from build123d import *

# Parameters (mm, degrees)
PAD017_DEPTH       = 15
SKETCH040_R        = 2
POCKET019_DEPTH    = 9.001
SKETCH_W           = 19.6
SKETCH_H           = 18.5
SKETCH_R           = 7.6
PAD_DEPTH          = 22
SKETCH002_W        = 17.1
SKETCH002_H        = 8.4
PAD001_DEPTH       = 8.5
POCKET_DEPTH       = 8
PAD002_DEPTH       = 13.6
SKETCH005_R        = 2
POCKET001_DEPTH    = 22.001
POCKET002_DEPTH    = 101.929968
POLARPATTERN_COUNT = 8
PAD004_DEPTH       = 1.5
SKETCH041_R        = 1.3
POCKET020_DEPTH    = 5


with BuildPart() as body023:
    # Sketch039 (on DatumPlane) → Pad017 (new body)
    with BuildSketch(Plane(origin=(0, -9.8, 0), x_dir=(0, 0, -1), z_dir=(0, -1, 0))):
        with BuildLine():
            Line((-9, 0), (-0.25, 0))
            Line((-0.25, 0), (-0.25, -6.907629))
            ThreePointArc((-0.25, -6.907629), (-4.1, -11), (-0.25, -15.092371))
            Line((-0.25, -15.092371), (-0.25, -22))
            Line((-0.25, -22), (-9, -22))
            Line((-9, -22), (-9, 0))
        make_face()
    extrude(amount=PAD017_DEPTH)

    # Sketch040 → Pocket019 (cut, through all)
    with BuildSketch(Plane.XY):
        with Locations((-18.546185, -20.8)):
            Circle(SKETCH040_R)
        with Locations((-18.546185, -13.8)):
            Circle(SKETCH040_R)
        with Locations((-3.453815, -13.8)):
            Circle(SKETCH040_R)
        with Locations((-3.453815, -20.8)):
            Circle(SKETCH040_R)
    extrude(amount=POCKET019_DEPTH, mode=Mode.SUBTRACT)


with BuildPart() as printable_axisholder_x_fusion:
    # Sketch → Pad (new body)
    with BuildSketch(Plane.YZ):
        with Locations((0, -0.25)):
            Rectangle(SKETCH_W, SKETCH_H)
        Circle(SKETCH_R, mode=Mode.SUBTRACT)
    extrude(amount=-PAD_DEPTH)

    # Sketch002 → Pad001 (join)
    with BuildSketch(Plane(origin=(0, 0, 9), x_dir=(0, -1, 0), z_dir=(0, 0, 1))):
        with Locations((-1.25, -17.8)):
            Rectangle(SKETCH002_W, SKETCH002_H)
    extrude(amount=PAD001_DEPTH)

    # Sketch003 → Pocket (cut)
    with BuildSketch(Plane(origin=(0, -7.3, 0), x_dir=(0, 0, -1), z_dir=(0, -1, 0))):
        with BuildLine():
            Line((-10.5, -22), (-10.5, -13.6))
            Line((-10.5, -13.6), (-11.6, -13.6))
            ThreePointArc((-12.1, -14.1), (-11.746447, -13.953553), (-11.6, -13.6))
            ThreePointArc((-12.1, -14.1), (-12.6, -14.6), (-12.1, -15.1))
            ThreePointArc((-12.1, -16.1), (-11.6, -15.6), (-12.1, -15.1))
            ThreePointArc((-12.1, -16.1), (-12.6, -16.6), (-12.1, -17.1))
            ThreePointArc((-12.1, -18.1), (-11.6, -17.6), (-12.1, -17.1))
            ThreePointArc((-12.1, -18.1), (-12.6, -18.6), (-12.1, -19.1))
            ThreePointArc((-12.1, -20.1), (-11.6, -19.6), (-12.1, -19.1))
            ThreePointArc((-12.1, -20.1), (-12.6, -20.6), (-12.1, -21.1))
            ThreePointArc((-11.8, -22), (-11.625658, -21.441886), (-12.1, -21.1))
            Line((-11.8, -22), (-10.5, -22))
        make_face()
    extrude(amount=-POCKET_DEPTH, mode=Mode.SUBTRACT)

    # Sketch004 (on DatumPlane) → Pad002 (join)
    with BuildSketch(Plane.YZ):
        Polygon((9.8, 17.5), (1.3, 17.5), (1.3, 16.25), (8.55, 16.25), (8.55, 9), (9.8, 9), align=None)
    extrude(amount=-PAD002_DEPTH)

    # Sketch005 (on DatumPlane) → Pocket001 (cut, through all)
    with BuildSketch(Plane.YZ):
        with Locations((4, 12.625)):
            Circle(SKETCH005_R)
    extrude(amount=-POCKET001_DEPTH, mode=Mode.SUBTRACT)

    # Sketch006 (on DatumPlane) → Pocket002 (cut, through all)
    with BuildSketch(Plane.YZ):
        with BuildLine():
            ThreePointArc((-7.846282, 1.560723), (-8, 0), (-7.846282, -1.560723))
            Line((-6.708571, -1.334418), (-7.846282, -1.560723))
            ThreePointArc((-6.708571, 1.334418), (-6.84, 0), (-6.708571, -1.334418))
            Line((-6.708571, 1.334418), (-7.846282, 1.560723))
        make_face()
    pocket002 = extrude(amount=-POCKET002_DEPTH, mode=Mode.SUBTRACT)

    # PolarPattern: Pocket002 ×8 about axis
    polarpattern_axis = Axis((0, 0, 0), (1, 0, 0))
    for i in range(1, POLARPATTERN_COUNT):
        add(pocket002.rotate(polarpattern_axis, i * 360 / POLARPATTERN_COUNT), mode=Mode.SUBTRACT)

    # Sketch010 (on DatumPlane) → Pad004 (join)
    with BuildSketch(Plane.XY.offset(9)):
        Polygon((0, -7.8), (-13.6, -7.8), (-13.6, -7.3), (-22, -7.3), (-22, -9.8), (0, -9.8), align=None)
    extrude(amount=PAD004_DEPTH)

    # Sketch041 → Pocket020 (cut)
    with BuildSketch(Plane.XY.offset(-9.5)):
        with Locations((-11, 0)):
            Circle(SKETCH041_R)
    extrude(amount=POCKET020_DEPTH, mode=Mode.SUBTRACT)

    # Fusion: union Body023
    add(body023.part)


solid = printable_axisholder_x_fusion.part
Work out the finished part from the listing and answer in its coordinate system (mm). A direction names the side the tool comes from. Coordinates: 2 decimals unless noted, no trailing zeros. Order: outer loops, then holes, each group sorted by start corner. A loop starts at its lowest first (then second) coordinate and runs counter-clockwise, first axis right, second up. Notation, with made-up numbers: (28.25, 23) - (41.25, 23) arc R33 cw to (41.25, 53) - close; hole circle Ø1 at (-11, 7.25). An arc over 180 degrees is marked (long way). Put each result on its own line as item: value. Start each with the question number.
1) Find the intervals of material crossed by line 1 (X direction, y = -20.8, z = 7); line 2 (Y direction, x = -11, z = -8.45); line 3 (Z direction, x = -16.75, y = 4) (3 decimals), in increasing order. Write a range as from..to.
2) Find section B-B (z = -3.75). Give the vertices of the cut face in (x, y).
3) Find section D-D (y = -17). Give the vertices of the cut face in (x, z).
4) For a pull along X with two mould halves and no side action, classify faces 4 (the cylindrical face through (-10.846, 7.013, -2.928)), 5 (the cylindrical face through (-10.9, -17.2, 4.1)) as released by +X, released by -X, zero draft, split by the parting line, or undercut.
5) For faces 1 (the flat face through (-7, 0, 9)), 2 (the cylindrical face through (-10.846, -7.013, 2.928)), 3 (the flat face through (-11, -24.8, 5)), determine the directions among +Z, -Z, +X, -X, +Y, -Y from which every point of the face is accessible in a straight line to the end or side of a thin tool.
6) Find section C-C (y = -5). Give the vertices of the cut face in (x, z) (3 decimals), plus the area to 3 significant figures.
7) Find section A-A (z = 3.5). Give the vertices of the cut face in (x, y).
8) Flat-ended cylindrical pins translate along their axes: pin 1 (3.5 mm diameter, centred on x = -3.45, y = -20.8, fed in from +Z) (3 decimals); pin 2 (5 mm diameter, centred on x = -9, y = -20.5, fed in from -Z); pin 3 (1.4 mm diameter, centred on x = -9, z = 17, fed in from -Y); pin 4 (4 mm diameter, centred on y = 0, z = 14, fed in from +X). Find the tip coordinate at first contact, or state that the pin passes through.
Results list:
1. line 1: x = -22..-20.55, -16.55..-5.45, -1.45..0
1. line 2: y = -9.8..-1.3, 1.3..9.8
1. line 3: z = -9.5..-6.462, 6.462..10.625, 14.625..17.5
2. outline: (-22, -9.8) - (0, -9.8) - (0, -6.61) - (-22, -6.61) - close; (-22, 6.61) - (0, 6.61) - (0, 9.8) - (-22, 9.8) - close
3. outline: (-22, 0.25) - (-15.09, 0.25) arc R4.1 cw to (-6.91, 0.25) - (0, 0.25) - (0, 9) - (-22, 9) - close
4. face 4: zero draft
4. face 5: undercut
5. face 1: +X
5. face 2: +X, -X
5. face 3: +Z, -Z, +X, -X, -Y
6. outline: (-22, -9.5) - (0, -9.5) - (0, -6.245) - (-22, -6.245) - close; (-22, 6.245) - (0, 6.245) - (0, 9) - (-13.6, 9) - (-13.6, 10.5) - (-22, 10.5) - close; (-22, 11.8) arc R0.5 ccw to (-21.1, 12.1) arc R0.5 cw to (-20.1, 12.1) arc R0.5 ccw to (-19.1, 12.1) arc R0.5 cw to (-18.1, 12.1) arc R0.5 ccw to (-17.1, 12.1) arc R0.5 cw to (-16.1, 12.1) arc R0.5 ccw to (-15.1, 12.1) arc R0.5 cw to (-14.1, 12.1) arc R0.5 ccw to (-13.6, 11.6) - (-13.6, 17.5) - (-22, 17.5) - close
6. area: 190 mm^2
7. outline: (-22, -24.8) - (-13.14, -24.8) - (-13.14, -9.8) - (-8.86, -9.8) - (-8.86, -24.8) - (0, -24.8) - (0, -6.75) - (-22, -6.75) - close; (-22, 6.75) - (0, 6.75) - (0, 9.8) - (-22, 9.8) - close; hole circle Ø4 at (-18.55, -20.8); hole circle Ø4 at (-18.55, -13.8); hole circle Ø4 at (-3.45, -20.8); hole circle Ø4 at (-3.45, -13.8)
8. pin 1: passes through
8. pin 2: stops at z = 0.25
8. pin 3: stops at y = 1.3
8. pin 4: stops at x = -13.6
